from build123d import *

# Parameters (mm, degrees)
SKETCH1_W           = 12.7
SKETCH1_H           = 12.7
BOSS_EXTRUDE1_DEPTH = 12.7
SKETCH2_R           = 3.55
CUT_EXTRUDE1_DEPTH  = 22.997045256
SKETCH3_R           = 3.55
CUT_EXTRUDE2_DEPTH  = 22.997045256
SKETCH4_R           = 3.55
CUT_EXTRUDE3_DEPTH  = 22.997045256


with BuildPart() as part:
    # Sketch1 → Boss-Extrude1 (new body)
    with BuildSketch(Plane(origin=(0, 0, 0), x_dir=(1, 0, 0), z_dir=(0, 1, 0))):
        with Locations((6.35, 6.35)):
            Rectangle(SKETCH1_W, SKETCH1_H)
    extrude(amount=BOSS_EXTRUDE1_DEPTH)

    # Sketch2 → Cut-Extrude1 (cut, through all)
    with BuildSketch(Plane(origin=(0, 12.7, 0), x_dir=(1, 0, 0), z_dir=(0, 1, 0))):
        with Locations(Location((6.35, 6.35, 0), (0, 0, 270))):
            Circle(SKETCH2_R)
    extrude(amount=-CUT_EXTRUDE1_DEPTH, mode=Mode.SUBTRACT)

    # Sketch3 → Cut-Extrude2 (cut, through all)
    with BuildSketch(Plane(origin=(12.7, 0, 0), x_dir=(0, 0, -1), z_dir=(1, 0, 0))):
        with Locations((6.35, 6.35)):
            Circle(SKETCH3_R)
    extrude(amount=-CUT_EXTRUDE2_DEPTH, mode=Mode.SUBTRACT)

    # Sketch4 → Cut-Extrude3 (cut, through all)
    with BuildSketch(Plane.XY):
        with Locations((6.35, 6.35)):
            Circle(SKETCH4_R)
    extrude(amount=-CUT_EXTRUDE3_DEPTH, mode=Mode.SUBTRACT)


solid = part.part
Part model, mm, in its own coordinate system. Coordinates: 2 decimals unless noted, no trailing zeros. Order: outer loops, then holes, each group sorted by start corner. A loop starts at its lowest first (then second) coordinate and runs counter-clockwise, first axis right, second up.
(1) Probe L1, parallel to Y at x = 6.35, z = -1.1; L2, parallel to Z at x = 6.35, y = 2.7. List the from-to ranges inside material, lowest first.
Check sheet entries:
L1: y = 0 to 2.8, 9.9 to 12.7
L2: z = -12.7 to -9.9, -2.8 to 0
(2) Slice it at B-B, the plane z = -6.35. Write the cut outline in (x, y).
Check sheet entries:
outline: (0, 0) - (2.8, 0) - (2.8, 2.8) - (0, 2.8) - close; (0, 9.9) - (2.8, 9.9) - (2.8, 12.7) - (0, 12.7) - close; (9.9, 0) - (12.7, 0) - (12.7, 2.8) - (9.9, 2.8) - close; (9.9, 9.9) - (12.7, 9.9) - (12.7, 12.7) - (9.9, 12.7) - close
(3) Pull direction Y, two halves, no side cores. Call faces 1 (the face through (3.734, 8.749, -11.18)), 2 (the face through (9, 3, -12.7)), 3 (the face through (9.1, 0, -3.6)), 4 (the face through (11.234, 8.749, -3.734)): pulls with the +Y half, pulls with the -Y half, needs draft (parallel to the pull), parting line crosses it, or undercut.
Check sheet entries:
face 1: undercut
face 2: needs draft
face 3: pulls with the -Y half
face 4: undercut
(4) Pin check, flat tip, straight feed: pin 1 Ø4.5 at (x, y) = (6.35, 6.35) entering from -Z. Stop position of the tip, or through.
Check sheet entries:
pin 1: passes through
(5) Slice it at C-C, the plane x = 2. Write the cut outline in (y, z).
Check sheet entries:
outline: (0, -12.7) - (12.7, -12.7) - (12.7, 0) - (0, 0) - close; hole circle Ø7.1 at (6.35, -6.35)
(6) Slice it at D-D, the plane z = -1. Write the cut outline in (x, y), and give its area (3 significant figures).
Check sheet entries:
outline: (0, 0) - (12.7, 0) - (12.7, 12.7) - (0, 12.7) - close; hole circle Ø7.1 at (6.35, 6.35)
area: 122 mm2
(7) Slice it at A-A, the plane y = 6.35. Write the cut outline in (x, z), and give its area (3 significant figures).
Check sheet entries:
outline: (0, -12.7) - (2.8, -12.7) - (2.8, -9.9) - (0, -9.9) - close; (0, -2.8) - (2.8, -2.8) - (2.8, 0) - (0, 0) - close; (9.9, -12.7) - (12.7, -12.7) - (12.7, -9.9) - (9.9, -9.9) - close; (9.9, -2.8) - (12.7, -2.8) - (12.7, 0) - (9.9, 0) - close
area: 31.4 mm2
